Geometry check sheet. Reference: the model listing, model coordinates, mm. A direction names the side the tool comes from. Give positions to 0.01 mm unless a question says otherwise; leave off trailing zeros. Loops run counter-clockwise (first coordinate to the right, second up) from the corner with the lowest first, then second, coordinate; pieces in that order, holes last. Notation, with made-up numbers: (49.25, 7.25) -> (77.25, 7.25) arc R12 cw to (77.25, 25.25) -> close; hole circle Ø8 at (-36.5, 44.25). An arc over 180 degrees is marked (long way). Answer in a Markdown table with one row per item. Add a question column.
```python
from build123d import *

# Parameters (mm, degrees)
F0_W     = 127
F0_H     = 19.05
F1_DEPTH = 76.2
F2_R     = 12.7
F3_DEPTH = 25.4
F5_DEPTH = 25.4


with BuildPart() as f1:
    # F0 (on Front) → F1 (new body)
    with BuildSketch(Plane.XZ):
        with Locations((3.121564, 23.662644)):
            Rectangle(F0_W, F0_H)
    extrude(amount=F1_DEPTH)

    # F2 (on face) → F3 (cut)
    with BuildSketch(Plane.XY.offset(33.187644)):
        with Locations((-22.278436, -38.1)):
            Circle(F2_R)
    extrude(amount=-F3_DEPTH, mode=Mode.SUBTRACT)

    # F4 (on face) → F5 (cut)
    with BuildSketch(Plane.XY.offset(33.187644)):
        Polygon((28.521564, -50.8), (15.821564, -28.802955), (3.121564, -50.8), align=None)
    extrude(amount=-F5_DEPTH, mode=Mode.SUBTRACT)


solid = f1.part
```
1. Release check for a two-part mould opening along X. For faces 3 (the face through (-60.378, -38, 24)), 4 (the face through (66.622, -38, 24)), 5 (the face through (-25.03, -50.5, 23.8)), 6 (the face through (16, -50.8, 24)) record: released by +X, released by -X, zero draft, split by the parting line, or undercut.
2. Sectioned sample at C-C (z = 22.5). Enter the section's corners in (x, y), plus the area to 3 significant figures.
3. Sectioned sample at D-D (y = -38.1). Enter the section's corners in (x, z), plus the area to 3 significant figures.
4. Access from +Z, -Z, +X, -X, +Y, -Y to the whole of each face (thin tool, end or side, straight path). Record for faces 1 (the face through (9.56, -39.65, 23.8)), 2 (the face through (2, -76.2, 24)).
5. Sectioned sample at B-B (x = 9.5). Enter the section's corners in (y, z).
6. Material ranges on L1, parallel to Y at x = -23, z = 27.25; L2, parallel to X at y = -42.5, z = 29.25 (3 decimals); L3, parallel to X at y = -48.5, z = 32, recorded low to high. Write a range as from..to.
7. Gauge pin test, flat end, axial feed: pin 1 Ø9.5 at (x, z) = (18, 26) entering from +Y. Record the tip position at first contact, or that the pin passes through.
8. Sectioned sample at A-A (y = -47). Enter the section's corners in (x, z), plus the area to 3 significant figures.
Response:
| question | item | result |
|---|---|---|
| 1 | face 3 | released by -X |
| 1 | face 4 | released by +X |
| 1 | face 5 | undercut |
| 1 | face 6 | undercut |
| 2 | outline | (-60.38, -76.2) -> (66.62, -76.2) -> (66.62, 0) -> (-60.38, 0) -> close; hole circle Ø25.4 at (-22.28, -38.1); hole (3.12, -50.8) -> (28.52, -50.8) -> (15.82, -28.8) -> close |
| 2 | area | 8,890 mm2 |
| 3 | outline | (-60.38, 14.14) -> (-34.98, 14.14) -> (-34.98, 33.19) -> (-60.38, 33.19) -> close; (-9.58, 14.14) -> (10.45, 14.14) -> (10.45, 33.19) -> (-9.58, 33.19) -> close; (21.19, 14.14) -> (66.62, 14.14) -> (66.62, 33.19) -> (21.19, 33.19) -> close |
| 3 | area | 1,730 mm2 |
| 4 | face 1 | +Z, -Z |
| 4 | face 2 | +Z, -Z, +X, -X, -Y |
| 5 | outline | (-76.2, 14.14) -> (-50.8, 14.14) -> (-50.8, 33.19) -> (-76.2, 33.19) -> close; (-39.75, 14.14) -> (0, 14.14) -> (0, 33.19) -> (-39.75, 33.19) -> close |
| 6 | L1 | y = -76.2..-50.78, -25.42..0 |
| 6 | L2 | x = -60.378..-34.192, -10.365..7.914, 23.73..66.622 |
| 6 | L3 | x = -60.38..-29.57, -14.99..4.45, 27.19..66.62 |
| 7 | pin 1 | stops at y = 0 |
| 8 | outline | (-60.38, 14.14) -> (-31.34, 14.14) -> (-31.34, 33.19) -> (-60.38, 33.19) -> close; (-13.22, 14.14) -> (5.32, 14.14) -> (5.32, 33.19) -> (-13.22, 33.19) -> close; (26.33, 14.14) -> (66.62, 14.14) -> (66.62, 33.19) -> (26.33, 33.19) -> close |
| 8 | area | 1,670 mm2 |
